```python
from build123d import *

# Parameters (mm, degrees)
SKETCH_W        = 11
SKETCH_H        = 20
PAD_DEPTH       = 15.2
POCKET001_DEPTH = 20
SKETCH008_W     = 13.6
SKETCH008_H     = 13.7
POCKET002_DEPTH = 11
POCKET003_DEPTH = 1.7
POCKET004_DEPTH = 1.7
SKETCH011_R     = 1
PAD001_DEPTH    = 1.5
FILLET_R        = 0.3
SKETCH012_R     = 1
PAD002_DEPTH    = 1.5
FILLET001_R     = 0.3
SKETCH013_W     = 11
SKETCH013_H     = 1.5
PAD003_DEPTH    = 25
SKETCH014_W     = 11
SKETCH014_H     = 1.5
PAD004_DEPTH    = 2
POCKET_DEPTH    = 11
POCKET005_DEPTH = 2


with BuildPart() as part:
    # Sketch → Pad (new body)
    with BuildSketch(Plane.XY):
        Rectangle(SKETCH_W, SKETCH_H)
    extrude(amount=PAD_DEPTH)

    # Sketch007 → Pocket001 (cut)
    with BuildSketch(Plane.XZ.offset(10)):
        with BuildLine():
            ThreePointArc((4.5, 10.20001), (-0.50001, 15.2), (-5.5, 10.19999))
            Line((-5.5, 10.19999), (-5.5, 16.2))
            Line((-5.5, 16.2), (5.5, 16.2))
            Line((5.5, 16.2), (5.5, 10.20001))
            Line((5.5, 10.20001), (4.5, 10.20001))
        make_face()
    extrude(amount=-POCKET001_DEPTH, mode=Mode.SUBTRACT)

    # Sketch008 (on Face7 of Pocket001) → Pocket002 (cut)
    with BuildSketch(Plane(origin=(-5.5, 0, 0), x_dir=(0, -1, 0), z_dir=(-1, 0, 0))):
        with Locations((0, 8.35)):
            Rectangle(SKETCH008_W, SKETCH008_H)
    extrude(amount=-POCKET002_DEPTH, mode=Mode.SUBTRACT)

    # Sketch009 (on Face8 of Pocket002) → Pocket003 (cut)
    with BuildSketch(Plane.XZ.offset(10)):
        with BuildLine():
            ThreePointArc((-0.49999, 4.7), (3.389081, 14.089094), (-6, 10.19999))
            Line((-6, 10.19999), (-6, 4.7))
            Line((-6, 4.7), (-0.49999, 4.7))
        make_face()
    extrude(amount=-POCKET003_DEPTH, mode=Mode.SUBTRACT)

    # Sketch010 (on Face1 of Pocket003) → Pocket004 (cut)
    with BuildSketch(Plane(origin=(0, 10, 0), x_dir=(-1, 0, 0), z_dir=(0, 1, 0))):
        with BuildLine():
            ThreePointArc((6, 10.19999), (-3.389081, 14.089094), (0.49999, 4.7))
            Line((0.49999, 4.7), (6, 4.7))
            Line((6, 4.7), (6, 10.19999))
        make_face()
    extrude(amount=-POCKET004_DEPTH, mode=Mode.SUBTRACT)

    # Sketch011 (on Face17 of Pocket004) → Pad001 (join)
    with BuildSketch(Plane.XZ.offset(8.3)):
        with Locations((-0.5, 10.2)):
            Circle(SKETCH011_R)
    extrude(amount=PAD001_DEPTH)

    # Fillet
    fillet_edges = [part.edges().sort_by_distance(p)[0] for p in [
        (-1.5, -9.8, 10.2),
    ]]
    fillet(fillet_edges, radius=FILLET_R)

    # Sketch012 (on Face15 of Fillet) → Pad002 (join)
    with BuildSketch(Plane(origin=(0, 8.3, 0), x_dir=(-1, 0, 0), z_dir=(0, 1, 0))):
        with Locations((0.5, 10.2)):
            Circle(SKETCH012_R)
    extrude(amount=PAD002_DEPTH)

    # Fillet001
    fillet001_edges = [part.edges().sort_by_distance(p)[0] for p in [
        (0.5, 9.8, 10.2),
    ]]
    fillet(fillet001_edges, radius=FILLET001_R)

    # Sketch013 (on Face20 of Fillet001) → Pad003 (join)
    with BuildSketch(Plane.XZ.offset(10)):
        with Locations((0, 0.75)):
            Rectangle(SKETCH013_W, SKETCH013_H)
    extrude(amount=PAD003_DEPTH)

    # Sketch014 (on Face11 of Pad003) → Pad004 (join)
    with BuildSketch(Plane(origin=(0, 10, 0), x_dir=(-1, 0, 0), z_dir=(0, 1, 0))):
        with Locations((0, 0.75)):
            Rectangle(SKETCH014_W, SKETCH014_H)
    extrude(amount=PAD004_DEPTH)

    # Sketch015 (on Face29 of Pad004) → Pocket (cut)
    with BuildSketch(Plane.XZ.offset(35)):
        Polygon((-4.15, 1.5), (-5.65, 0), (-5.65, 2.5), (5.65, 2.5), (5.65, 0), (4.15, 1.5), align=None)
    extrude(amount=-POCKET_DEPTH, mode=Mode.SUBTRACT)

    # Sketch016 (on Face33 of Pocket) → Pocket005 (cut)
    with BuildSketch(Plane(origin=(0, 12, 0), x_dir=(-1, 0, 0), z_dir=(0, 1, 0))):
        Polygon((-4.15, 1.5), (-5.65, 0), (-5.65, 2.5), (5.65, 2.5), (5.65, 0), (4.15, 1.5), align=None)
    extrude(amount=-POCKET005_DEPTH, mode=Mode.SUBTRACT)


solid = part.part
```
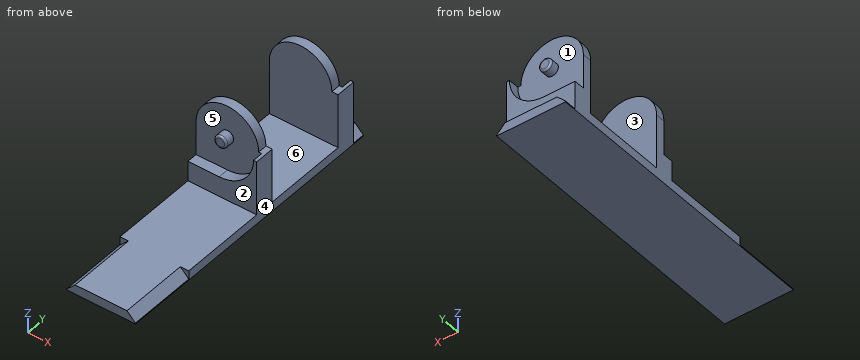
Geometry check sheet. Reference: the model listing, model coordinates, mm. Face numbers are marked on the shaded views. A direction names the side the tool comes from. Coordinates: 2 decimals unless noted, no trailing zeros. Order: outer loops, then holes, each group sorted by start corner. A loop starts at its lowest first (then second) coordinate and runs counter-clockwise, first axis right, second up.
Item 1: Tool access check on the marked faces 1, 2 and 3. Record the directions out of +Z, -Z, +X, -X, +Y, -Y that give a thin tool (end or side, any length) a straight path to the whole face; none if there is none.
Item 2: Section check D-D (y = -19.5). Enter the section's corners in (x, z).
Item 3: Scan lines: line 1 along Y through (x, z) = (-2.5, 2.75); line 2 along Y through (x, z) = (0.5, 8); line 3 along Z through (x, y) = (2, -32.5). Record each from-to range of solid material in increasing order.
Item 4: Section check B-B (y = 7.5). Enter the section's corners in (x, z), plus the area to 3 significant figures.
Item 5: Depth check by flat-ended pin: pin 1 (3.5 mm diameter, centred on x = 1, z = 7.5, fed in from -Y); pin 2 (3.5 mm diameter, centred on x = -1.5, y = -24.5, fed in from +Z); pin 3 (1.9 mm diameter, centred on x = -3, y = -9, fed in from +Z); pin 4 (3 mm diameter, centred on x = 1, y = -14.5, fed in from -Z). Enter the tip coordinate at first touch or a pass-through.
Item 6: Mould release check, pull along Y, two halves, no side actions. Record for the marked faces 4, 5 and 6: released by +Y, released by -Y, zero draft, split by the parting line, or undercut.
Item 7: Section check A-A (z = 13.25). Enter the section's corners in (x, y), plus the area to 3 significant figures.
Item 8: Section check C-C (x = -3). Enter the section's corners in (y, z), plus the area to 3 significant figures.
Check sheet entries:
1. face 1: +Y
1. face 2: +Z, +X, -X, -Y
1. face 3: +Z, +X, -X
2. outline: (-5.5, 0) - (5.5, 0) - (5.5, 1.5) - (-5.5, 1.5) - close
3. line 1: y = -10 to -6.8, 6.8 to 10
3. line 2: y = -8.3 to -6.8, 6.8 to 8.3
3. line 3: z = 0 to 1.5
4. outline: (-5.5, 0) - (5.5, 0) - (5.5, 10.2) - (4.5, 10.2) arc R5 ccw to (-5.5, 10.2) - close
4. area: 151 mm2
5. pin 1: stops at y = -8.3
5. pin 2: stops at z = 1.5
5. pin 3: stops at z = 14.84
5. pin 4: stops at z = 0
6. face 4: zero draft
6. face 5: released by -Y
6. face 6: undercut
7. outline: (-4.46, -8.3) - (3.46, -8.3) - (3.46, -6.8) - (-4.46, -6.8) - close; (-4.46, 6.8) - (3.46, 6.8) - (3.46, 8.3) - (-4.46, 8.3) - close
7. area: 23.8 mm2
8. outline: (-35, 0) - (12, 0) - (12, 1.5) - (10, 1.5) - (10, 4.7) - (8.3, 4.7) - (8.3, 14.53) - (6.8, 14.53) - (6.8, 1.5) - (-6.8, 1.5) - (-6.8, 14.53) - (-8.3, 14.53) - (-8.3, 4.7) - (-10, 4.7) - (-10, 1.5) - (-35, 1.5) - close
8. area: 120 mm2
